from build123d import *

# Parameters (mm, degrees)
F1_DEPTH = 8
F3_DEPTH = 2.4
F2_W     = 18
F2_H     = 8
F5_DEPTH = 2.4
F7_DEPTH = 25
F8_R     = 1.6
F9_DEPTH = 25
F10_R    = 4


with BuildPart() as f1:
    # F0 (on Front) → F1 (new body)
    with BuildSketch(Plane.XZ):
        Polygon((-11.162, 13.4169430507), (-11.162, 14.9166165667), (-12.1126689762, 14.4412820786), (-12.1126689762, 13.8922775388), align=None)
        Polygon((-11.162, 11.8669430507), (-11.162, 13.3666165667), (-12.1126689762, 12.8912820786), (-12.1126689762, 12.3422775388), align=None)
        Polygon((-9, 7.217), (-9, 15), (-11.162, 15), (-11.162, 14.9166165667), (-11.162, 13.4169430507), (-11.162, 13.3666165667), (-11.162, 11.8669430507), (-11.162, 11.8166165667), (-11.162, 10.3169430507), (-11.162, 10.2666165667), (-11.162, 8.7669430507), (-11.162, 8.7166165667), (-11.162, 7.217), align=None)
        with BuildLine():
            ThreePointArc((9, -11), (3.0408534236, 2.4778498939), (-4.728292115, 15))
            Line((-4.728292115, 15), (-9, 15))
            Line((-9, 15), (-9, 7.217))
            Line((-9, 7.217), (-9, 7))
            ThreePointArc((-9, 7), (-6.8605710995, -2), (-9, -11))
            Line((-9, -11), (9, -11))
        make_face()
        Polygon((-12.1126689762, 10.7922775388), (-11.162, 10.3169430507), (-11.162, 11.8166165667), (-12.1126689762, 11.3412820786), align=None)
        Polygon((-12.1126689762, 9.2422775388), (-11.162, 8.7669430507), (-11.162, 10.2666165667), (-12.1126689762, 9.7912820786), align=None)
        Polygon((-12.1126689762, 7.6923344881), (-11.162, 7.217), (-11.162, 8.7166165667), (-12.1126689762, 8.2412820786), align=None)
        Polygon((9, -15), (9, -11), (-9, -11), (-9, -15), (-9, -19), (9, -19), align=None)
    extrude(amount=-F1_DEPTH)

    # F0 (on Front) → F3 (cut)
    with BuildSketch(Plane.XZ):
        Polygon((9, -15), (9, -11), (-9, -11), (-9, -15), (-9, -19), (9, -19), align=None)
    extrude(amount=-F3_DEPTH, mode=Mode.SUBTRACT)

    # F2 (on face) → F5 (cut)
    with BuildSketch(Plane(origin=(0, 8, 0), x_dir=(-1, 0, 0), z_dir=(0, 1, 0))):
        with Locations((0, -15)):
            Rectangle(F2_W, F2_H)
    extrude(amount=-F5_DEPTH, mode=Mode.SUBTRACT)

    # F6 (on face) → F7 (cut)
    with BuildSketch(Plane.XZ):
        with BuildLine():
            ThreePointArc((4.6301934316, -8), (-0.1534331268, 2.0887492698), (-6, 11.6010360967))
            Line((-6, 11.6010360967), (-6, 7.6869279652))
            ThreePointArc((-6, 7.6869279652), (-3.9444041717, -0.038038396), (-4.6569677883, -8))
            Line((-4.6569677883, -8), (4.6301934316, -8))
        make_face()
    extrude(amount=-F7_DEPTH, mode=Mode.SUBTRACT)

    # F8 (on face) → F9 (cut)
    with BuildSketch(Plane.XZ.offset(-2.4)):
        with Locations((-4.6, -15.6)):
            Circle(F8_R)
        with Locations((4.7, -15.6)):
            Circle(F8_R)
    extrude(amount=-F9_DEPTH, mode=Mode.SUBTRACT)

    # F10
    f10_edges = [f1.edges().sort_by_distance(p)[0] for p in [
        (-9, 4, -19),
        (9, 4, -19),
    ]]
    fillet(f10_edges, radius=F10_R)


solid = f1.part
Verification items for the finished model (mm, model axes). A direction names the side the tool comes from. Coordinates: 2 decimals unless noted, no trailing zeros. Loops run counter-clockwise (first coordinate to the right, second up) from the corner with the lowest first, then second, coordinate; pieces in that order, holes last. Notation, with made-up numbers: (70.5, 29.5) -> (115.5, 29.5) arc R18 ccw to (115.5, 64.5) -> close; hole circle Ø9 at (88, -37). An arc over 180 degrees is marked (long way). Answer as a JSON object with one key per item and string values. Group by question number.
Item 1: Scan lines: probe 1 along X at (y, z) = (6.25, 4.5); probe 2 along Z at (x, y) = (4.7, 4.7); probe 3 along X at (y, z) = (3, -3.5). Record each from-to range of solid material in increasing order.
Item 2: Depth check by flat-ended pin: pin 1 (3.5 mm diameter, centred on x = 4.7, z = -15.6, fed in from +Y); pin 2 (1 mm diameter, centred on y = 6.5, z = -7, fed in from -X); pin 3 (3 mm diameter, centred on y = 4, z = 9.5, fed in from +X). Enter the tip coordinate at first touch or a pass-through.
Item 3: Sectioned sample at C-C on z = -1.5. Record the boundary of the cut face in (x, y).
Item 4: Sectioned sample at D-D on x = 0.75. Record the boundary of the cut face in (y, z), plus the area to 3 significant figures.
Item 5: Sectioned sample at A-A on z = -15.6. Record the boundary of the cut face in (x, y), plus the area to 3 significant figures.
Item 6: Sectioned sample at B-B on x = -5.5. Record the boundary of the cut face in (y, z), plus the area to 3 significant figures.
Item 7: Tool access check on faces 4 (the flat face through (-9, 4, -13)), 5 (the flat face through (-11.644, 3.944, 10.558)), 6 (the flat face through (0, 7, -11)). Record the directions out of +Z, -Z, +X, -X, +Y, -Y that give a thin tool (end or side, any length) a straight path to the whole face; none if there is none.
Item 8: Mould release check, pull along X, two halves, no side actions. Record for faces 1 (the flat face through (-11.631, 3.944, 11.582)), 2 (the flat face through (0, 2.4, -15)), 3 (the cylindrical face through (-0.08, 3.94, 1.95)): +X half, -X half, draft (parallel to the pull), parting line (faces both ways), or undercut.
Evaluation:
{
 "1": {"probe 1": "x = -7.95 to -4.8, -1.5 to 1.94", "probe 2": "z = -19 to -17.2, -14 to -0.8", "probe 3": "x = -6.92 to -3.91, 2.66 to 5.96"},
 "2": {"pin 1": "stops at y = 5.6", "pin 2": "stops at x = -7.63", "pin 3": "stops at x = -0.09"},
 "3": {"outline": "(-6.87, 0) -> (-3.87, 0) -> (-3.87, 8) -> (-6.87, 8) -> close; (1.7, 0) -> (5.04, 0) -> (5.04, 8) -> (1.7, 8) -> close"},
 "4": {"outline": "(0, -11) -> (2.4, -11) -> (2.4, -19) -> (5.6, -19) -> (5.6, -11) -> (8, -11) -> (8, -8) -> (0, -8) -> close; (0, 0.39) -> (8, 0.39) -> (8, 6.59) -> (0, 6.59) -> close", "area": "99.3 mm²"},
 "5": {"outline": "(-8.95, 2.4) -> (-6.2, 2.4) -> (-6.2, 5.6) -> (-8.95, 5.6) -> close; (-3, 2.4) -> (3.1, 2.4) -> (3.1, 5.6) -> (-3, 5.6) -> close; (6.3, 2.4) -> (8.95, 2.4) -> (8.95, 5.6) -> (6.3, 5.6) -> close", "area": "36.8 mm²"},
 "6": {"outline": "(0, -11) -> (2.4, -11) -> (2.4, -14.28) -> (5.6, -14.28) -> (5.6, -11) -> (8, -11) -> (8, 6.53) -> (0, 6.53) -> close; (0, 10.87) -> (8, 10.87) -> (8, 15) -> (0, 15) -> close; (2.4, -18.97) -> (5.6, -18.97) -> (5.6, -16.92) -> (2.4, -16.92) -> close", "area": "190 mm²"},
 "7": {"face 4": "-Z, -X, +Y, -Y", "face 5": "-X, +Y, -Y", "face 6": "-Z, +X, -X, +Y"},
 "8": {"face 1": "-X half", "face 2": "draft", "face 3": "undercut"}
}
